```python
from build123d import *

# Parameters (mm, degrees)
FORCAD_DEPTH = 609.6
FILLET1_R    = 101.6


with BuildPart() as part:
    # Sketch1 → ForCAD (new body)
    with BuildSketch(Plane(origin=(0, 0, 0), x_dir=(1, 0, 0), z_dir=(0, 1, 0))):
        Polygon((0, 0), (225.091665708, 32.392093885), (314.955840223, 14.435459902), (315.266904727, 15.992185673), (225.135389647, 34.002239572), (-0.226121766, 1.571313208), align=None)
    extrude(amount=FORCAD_DEPTH)

    # Fillet1
    fillet1_edges = [part.edges().sort_by_distance(p)[0] for p in [
        (225.135389647, 304.8, -34.002239572),
        (225.091665708, 304.8, -32.392093885),
    ]]
    fillet(fillet1_edges, radius=FILLET1_R)


solid = part.part
```
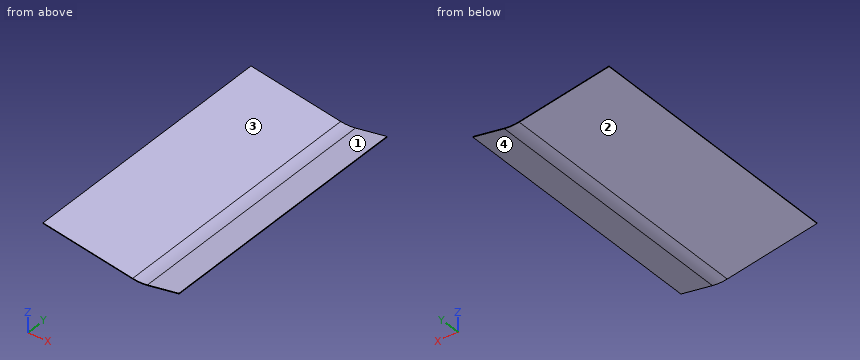
The model under review builds one solid part; all positions refer to its coordinate system, in mm. Face numbers are marked on the shaded views. Round coordinates to 2 decimals unless told otherwise and drop trailing zeros. Order: outer loops, then holes, each group sorted by start corner. A loop starts at its lowest first (then second) coordinate and runs counter-clockwise, first axis right, second up.
(1) Take a section at B-B, the plane y = 340.5. State the section outline as (x, z) points, plus the area to 3 significant figures.
Working result:
outline: (-0.23, -1.57) - (207.87, -31.52) arc R101.6 ccw to (242.25, -30.58) - (315.27, -15.99) - (314.96, -14.44) - (242.2, -28.97) arc R101.6 cw to (207.82, -29.91) - (0, 0) - close
area: 507 mm2
(2) Take a section at D-D, the plane x = 273. State the section outline as (y, z) points.
Working result:
outline: (0, -24.44) - (609.6, -24.44) - (609.6, -22.82) - (0, -22.82) - close
(3) Take a section at A-A, the plane z = -21. State the section outline as (x, y) points, plus the area to 3 significant figures.
Working result:
outline: (134.78, 0) - (145.93, 0) - (145.93, 609.6) - (134.78, 609.6) - close; (282.1, 0) - (290.21, 0) - (290.21, 609.6) - (282.1, 609.6) - close
area: 11,700 mm2
(4) Mouldability with a two-part tool opening along X and no side actions: class the marked faces 1, 2, 3 and 4 as released by +X, released by -X, zero draft, split by the parting line, or undercut.
Working result:
face 1: undercut
face 2: released by -X
face 3: undercut
face 4: released by +X
(5) Wall thickness on L1, parallel to Z at x = 232, y = 99; L2, parallel to Z at x = 36, y = 532: over which ranges is each line inside the solid? List them lowest first.
Working result:
L1: z = -32.09 to -30.48
L2: z = -6.78 to -5.18
(6) Take a section at C-C, the plane x = 99. State the section outline as (y, z) points, plus the area to 3 significant figures.
Working result:
outline: (0, -15.85) - (609.6, -15.85) - (609.6, -14.25) - (0, -14.25) - close
area: 978 mm2
(7) For P1, Ø1.5, axis at x = 234, y = 148.5, coming from the -Z side; P2, Ø4, axis at x = 103.5, z = -11, coming from the +Y side; P3, Ø1, axis at x = 48, y = 345.5, coming from the -Z side; P4, Ø1.5, axis at x = 41.5, y = 132.5, coming from the +Z side, all flat-tipped, find the tip position at first contact; note any pin that passes through.
Working result:
P1: stops at z = -31.97
P2: passes through
P3: stops at z = -8.58
P4: stops at z = -5.86
